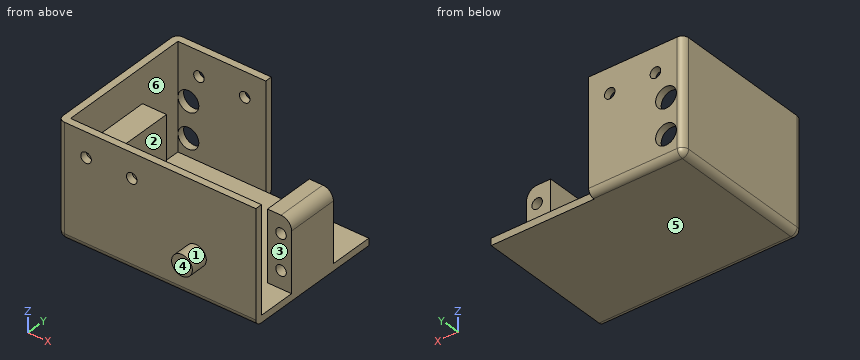
from build123d import *

# Parameters (mm, degrees)
SKETCH_W        = 54.3
SKETCH_H        = 38.5
PAD_DEPTH       = 2
SKETCH003_W     = 6.85
SKETCH003_H     = 15
PAD001_DEPTH    = 20
SKETCH001_W     = 54.3
SKETCH001_H     = 2
PAD003_DEPTH    = 32
SKETCH005_W     = 6.85
SKETCH005_H     = 15
PAD004_DEPTH    = 20
SKETCH002_R     = 2.95
PAD005_DEPTH    = 5
SKETCH007_W     = 25
SKETCH007_H     = 32
PAD006_DEPTH    = 2
SKETCH006_R     = 1.5
POCKET_DEPTH    = 15
SKETCH004_R     = 1.5
POCKET001_DEPTH = 20
SKETCH009_R     = 1.5
SKETCH009_R_2   = 2.95
POCKET002_DEPTH = 2
SKETCH008_R     = 1.5
POCKET003_DEPTH = 3
SKETCH010_W     = 42.5
SKETCH010_H     = 32
PAD007_DEPTH    = 2
FILLET_R        = 1.8
FILLET001_R     = 1.8
FILLET002_R     = 1.8
FILLET003_R     = 3


with BuildPart() as part:
    # Sketch → Pad (new body)
    with BuildSketch(Plane.XY):
        with Locations((27.15, 21.25)):
            Rectangle(SKETCH_W, SKETCH_H)
    extrude(amount=PAD_DEPTH)

    # Sketch003 → Pad001 (join)
    with BuildSketch(Plane.XY.offset(2)):
        with Locations((3.425, 20.3)):
            Rectangle(SKETCH003_W, SKETCH003_H)
    extrude(amount=PAD001_DEPTH)

    # Sketch001 → Pad003 (join)
    with BuildSketch(Plane.XY):
        with Locations((27.15, 1)):
            Rectangle(SKETCH001_W, SKETCH001_H)
    extrude(amount=PAD003_DEPTH)

    # Sketch005 (on Face5 of Pad003) → Pad004 (join)
    with BuildSketch(Plane.XY.offset(2)):
        with Locations((50.875, 20.3)):
            Rectangle(SKETCH005_W, SKETCH005_H)
    extrude(amount=PAD004_DEPTH)

    # Sketch002 (on Face18 of Pad004) → Pad005 (join)
    with BuildSketch(Plane.XZ):
        with Locations((37.25, 12)):
            Circle(SKETCH002_R)
    extrude(amount=PAD005_DEPTH)

    # Sketch007 (on Face1 of Pad005) → Pad006 (join)
    with BuildSketch(Plane(origin=(0, 40.5, 0), x_dir=(-1, 0, 0), z_dir=(0, 1, 0))):
        with Locations((-12.5, 16)):
            Rectangle(SKETCH007_W, SKETCH007_H)
    extrude(amount=PAD006_DEPTH)

    # Sketch006 (on Face14 of Pad006) → Pocket (cut)
    with BuildSketch(Plane.XZ.offset(-12.8)):
        with Locations((51.3, 17)):
            Circle(SKETCH006_R)
        with Locations((51.3, 7)):
            Circle(SKETCH006_R)
    extrude(amount=-POCKET_DEPTH, mode=Mode.SUBTRACT)

    # Sketch004 (on Face16 of Pocket) → Pocket001 (cut)
    with BuildSketch(Plane.XZ.offset(-12.8)):
        with Locations((3, 17)):
            Circle(SKETCH004_R)
        with Locations((3, 7)):
            Circle(SKETCH004_R)
    extrude(amount=-POCKET001_DEPTH, mode=Mode.SUBTRACT)

    # Sketch009 (on Face20 of Pocket001) → Pocket002 (cut)
    with BuildSketch(Plane(origin=(0, 42.5, 0), x_dir=(-1, 0, 0), z_dir=(0, 1, 0))):
        with Locations((-6, 25)):
            Circle(SKETCH009_R)
        with Locations((-19, 25)):
            Circle(SKETCH009_R)
        with Locations((-3, 7)):
            Circle(SKETCH009_R_2)
        with Locations((-3, 17)):
            Circle(SKETCH009_R_2)
    extrude(amount=-POCKET002_DEPTH, mode=Mode.SUBTRACT)

    # Sketch008 → Pocket003 (cut)
    with BuildSketch(Plane.XZ):
        with Locations((19, 25)):
            Circle(SKETCH008_R)
        with Locations((6, 25)):
            Circle(SKETCH008_R)
    extrude(amount=-POCKET003_DEPTH, mode=Mode.SUBTRACT)

    # Sketch010 (on Face8 of Pocket003) → Pad007 (join)
    with BuildSketch(Plane(origin=(0, 0, 0), x_dir=(0, -1, 0), z_dir=(-1, 0, 0))):
        with Locations((-21.25, 16)):
            Rectangle(SKETCH010_W, SKETCH010_H)
    extrude(amount=PAD007_DEPTH)

    # Fillet
    fillet_edges = [part.edges().sort_by_distance(p)[0] for p in [
        (-2, 42.5, 16),
    ]]
    fillet(fillet_edges, radius=FILLET_R)

    # Fillet001
    fillet001_edges = [part.edges().sort_by_distance(p)[0] for p in [
        (-2, 0, 16),
    ]]
    fillet(fillet001_edges, radius=FILLET001_R)

    # Fillet002
    fillet002_edges = [part.edges().sort_by_distance(p)[0] for p in [
        (-2, 21.25, 0),
    ]]
    fillet(fillet002_edges, radius=FILLET002_R)

    # Fillet003
    fillet003_edges = [part.edges().sort_by_distance(p)[0] for p in [
        (54.3, 20.3, 22),
    ]]
    fillet(fillet003_edges, radius=FILLET003_R)


solid = part.part
The listing builds one solid part. Answer for the finished solid, in the listing's coordinates (mm). Face numbers are marked on the shaded views. A direction names the side the tool comes from. Coordinates: 2 decimals unless noted, no trailing zeros. Write each loop counter-clockwise with the first axis right and the second up, starting at its lowest first coordinate (ties: lowest second). Pieces come first, ordered by that corner, then holes. Notation, with made-up numbers: M -12,34 L 32,34 A19 cw 32,65 Z; hole C 88.5,44 d3. An arc over 180 degrees is marked long. Put each result on its own line as item: value. Start each with the question number.
1. A cutting plane is placed at A-A on y = 24. Write down the section's boundary in (x, z), then the cut area to 3 significant figures.
2. A cutting plane is placed at B-B on z = 12. Write down the section's boundary in (x, y).
3. A cutting plane is placed at C-C on x = 3. Count the separate pieces of the cut face and the enclosed holes in it, then the cut area to 3 significant figures.
4. For a pull along Y with two mould halves and no side action, classify the marked faces 4, 5 and 6 as pulls with the +Y half, pulls with the -Y half, needs draft (parallel to the pull), parting line crosses it, or undercut.
5. Consider line 1 (Z direction, x = 51.3, y = 24.75); line 2 (Y direction, x = 2, z = 3.5); line 3 (Y direction, x = 51, z = 14). Determine where each line is inside the solid, lowest interval first. Write a range as from..to.
6. Which of the six approach directions +Z, -Z, +X, -X, +Y, -Y give full straight-line access (tool end or side, diameter ignored) to the marked faces 1, 2 and 3?
7. Flat-ended cylindrical pins translate along their axes: P1, Ø2.5, axis at x = 51.3, z = 17, coming from the +Y side; P2, Ø5.5, axis at x = 3, z = 7, coming from the +Y side; P3, Ø3, axis at x = 46, y = 33.5, coming from the +Z side; P4, Ø2.5, axis at x = 6, z = 25, coming from the +Y side (3 decimals). Find the tip coordinate at first contact, or state that the pin passes through.
Resolved:
1. outline: M -2,1.8 A1.8 ccw -0.2,0 L 54.3,0 L 54.3,19 A3 ccw 51.3,22 L 47.45,22 L 47.45,2 L 6.85,2 L 6.85,22 L 0,22 L 0,32 L -2,32 Z; hole C 3,7 d3; hole C 3,17 d3; hole C 51.3,7 d3; hole C 51.3,17 d3
1. area: 416 mm2
2. outline: M -2,1.8 A1.8 ccw -0.2,0 L 34.3,0 L 34.3,-5 L 40.2,-5 L 40.2,0 L 54.3,0 L 54.3,2 L 0,2 L 0,12.8 L 6.85,12.8 L 6.85,27.8 L 0,27.8 L 0,40.5 L 25,40.5 L 25,42.5 L -0.2,42.5 A1.8 ccw -2,40.7 Z; M 47.45,12.8 L 54.3,12.8 L 54.3,27.8 L 47.45,27.8 Z
3. separate pieces: 5
3. enclosed holes: 0
3. area: 390 mm2
4. face 4: pulls with the -Y half
4. face 5: needs draft
4. face 6: undercut
5. line 1: z = 0..5.5, 8.5..15.5, 18.5..22
5. line 2: y = 0..2, 12.8..27.8, 40.5..42.5
5. line 3: y = 0..2, 12.8..27.8
6. face 1: -Y
6. face 2: +Z
6. face 3: +Z, +X
7. P1: stops at y = 2
7. P2: stops at y = 27.8
7. P3: stops at z = 2
7. P4: passes through
